Build history of the part. All positions in model axes, mm. Give positions to 0.01 mm unless a question says otherwise; leave off trailing zeros. Loops run counter-clockwise (first coordinate to the right, second up) from the corner with the lowest first, then second, coordinate; pieces in that order, holes last. Notation, with made-up numbers: M 80.5,13.25 L 126.5,13.25 A17 ccw 126.5,32.25 Z; hole C 55.5,46 d3. An arc over 180 degrees is marked long. Answer as a JSON object with one key per item and string values. Group by question number.
1. Slice it at A-A (x = 49). List the corners of the cut face in (y, z), then the cut area to 3 significant figures.
2. Drill centre lines: line 1 along Y through (x, z) = (73, 1610); line 2 along Z through (x, y) = (33.5, 89); line 3 along Z through (x, y) = (91.5, 180.5). Where is each one in solid material? Low to high. Write a range as [from, to].
3. Drop flat-ended pins along their axis: pin 1 Ø22 at (y, z) = (48, 1710) entering from +X; pin 2 Ø10 at (x, y) = (158, 83) entering from +Z. Give the stop position or say it passes through.
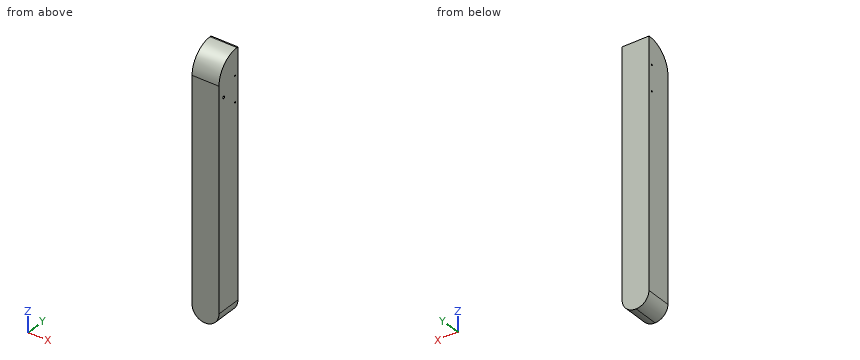
from build123d import *

# Parameters (mm, degrees)
SKETCH1_W           = 210
SKETCH1_H           = 2010
BOSS_EXTRUDE1_DEPTH = 200
FILLET1_R           = 110
FILLET2_R           = 100
FILLET3_R           = 190
SKETCH3_R           = 10
CUT_EXTRUDE1_DEPTH  = 10
SKETCH4_R           = 5
CUT_EXTRUDE2_DEPTH  = 2031.812645224


with BuildPart() as part:
    # Sketch1 → Boss-Extrude1 (new body)
    with BuildSketch(Plane(origin=(0, 0, 0), x_dir=(1, 0, 0), z_dir=(0, 1, 0))):
        with Locations((105, -1005)):
            Rectangle(SKETCH1_W, SKETCH1_H)
    extrude(amount=BOSS_EXTRUDE1_DEPTH)

    # Fillet1
    fillet1_edges = [part.edges().sort_by_distance(p)[0] for p in [
        (210, 100, 0),
    ]]
    fillet(fillet1_edges, radius=FILLET1_R)

    # Fillet2
    fillet2_edges = [part.edges().sort_by_distance(p)[0] for p in [
        (0, 100, 0),
    ]]
    fillet(fillet2_edges, radius=FILLET2_R - 0.0001)  # a hair under: the kernel refuses the full size

    # Fillet3
    fillet3_edges = [part.edges().sort_by_distance(p)[0] for p in [
        (105, 0, 2010),
    ]]
    fillet(fillet3_edges, radius=FILLET3_R)

    # Sketch3 → Cut-Extrude1 (cut)
    with BuildSketch(Plane(origin=(210, 0, 0), x_dir=(0, 0, -1), z_dir=(1, 0, 0))):
        with Locations((-1710, 50)):
            Circle(SKETCH3_R)
    extrude(amount=-CUT_EXTRUDE1_DEPTH, mode=Mode.SUBTRACT)

    # Sketch4 → Cut-Extrude2 (cut, through all)
    with BuildSketch(Plane(origin=(210, 0, 0), x_dir=(0, 0, -1), z_dir=(1, 0, 0))):
        with Locations((-1810, 170)):
            Circle(SKETCH4_R)
        with Locations((-1610, 170)):
            Circle(SKETCH4_R)
    extrude(amount=-CUT_EXTRUDE2_DEPTH, mode=Mode.SUBTRACT)


solid = part.part
Established:
{
 "1": {"outline": "M 0,13.98 L 200,13.98 L 200,2010 L 190,2010 A190 ccw 0,1820 Z; hole C 170,1610 d10; hole C 170,1810 d10", "area": "391,000 mm^2"},
 "2": {"line 1": "y = [0, 165], [175, 200]", "line 2": "z = [25.32, 1980.93]", "line 3": "z = [0.36, 2009.76]"},
 "3": {"pin 1": "stops at x = 210", "pin 2": "stops at z = 1980.3"}
}
